from build123d import *

# Parameters (mm, degrees)
EXTRUDE_START   = -3.875
SKETCH_1_R      = 2.225
EXTRUDE_1_DEPTH = 1.6
SKETCH_1_3_R    = 4.255
SKETCH_1_3_R_2  = 2.225
EXTRUDE_2_DEPTH = 3.875


with BuildPart() as part:
    # Эскиз1 → Бобышка-Вытянуть1 (new body)
    with BuildSketch(Plane.XY.offset(EXTRUDE_START)):
        with BuildLine():
            Line((0, 4.045727726), (0, -4.045727726))
            ThreePointArc((0, -4.045727726), (-1.653799143, -4.282252786), (-3.175, -4.972863863))
            ThreePointArc((-3.175, -4.972863863), (-12.25, 0), (-3.175, 4.972863863))
            ThreePointArc((-3.175, 4.972863863), (-1.653799143, 4.282252786), (0, 4.045727726))
        make_face()
        with Locations((-6.35, 0)):
            Circle(SKETCH_1_R, mode=Mode.SUBTRACT)
    extrude(amount=-EXTRUDE_1_DEPTH)

    # Эскиз1<3> → Бобышка-Вытянуть2 (add)
    with BuildSketch(Plane.XY):
        with Locations((-6.35, 0)):
            Circle(SKETCH_1_3_R)
        with Locations((-6.35, 0)):
            Circle(SKETCH_1_3_R_2, mode=Mode.SUBTRACT)
    extrude(amount=-EXTRUDE_2_DEPTH)

    # Зеркальное отражение1: part across plane


with BuildPart() as part_1:
    add(part.part)
    add(part.part.mirror(Plane(origin=(0, 0, 0), x_dir=(0, 0, 1), z_dir=(1, 0, 0))))

    # Зеркальное отражение2: part across plane


with BuildPart() as part_2:
    add(part_1.part)
    add(part_1.part.mirror(Plane.XY))


solid = part_2.part
Geometry: final body of the model. Coordinates: model frame, mm. A direction names the side the tool comes from. Give positions to 0.01 mm unless a question says otherwise; leave off trailing zeros. Write each loop counter-clockwise with the first axis right and the second up, starting at its lowest first coordinate (ties: lowest second). Pieces come first, ordered by that corner, then holes. Notation, with made-up numbers: (-14, 72) - (4, 72) arc R34 cw to (4, 109) - close; hole circle Ø7 at (26.5, 5.25). An arc over 180 degrees is marked (long way). Return JSON: item names as keys, results as strings. Group by question number.
1) Section C-C on z = -0.25. Return the cut outline in (x, y) (3 decimals).
2) Section D-D on y = -2.5. Return the cut outline in (x, z) (3 decimals), plus the area to 3 significant figures.
3) Line query: line 1 (Z direction, x = 3, y = -4.75) (3 decimals); line 2 (Y direction, x = 6.35, z = -0.25) (3 decimals); line 3 (X direction, y = 1.75, z = -2.5). Output: solid intervals per line, ascending.
4) First-contact query: P1, Ø1, axis at x = -2, z = 2, coming from the -Y side; P2, Ø3.5, axis at x = -6.35, y = 0, coming from the -Z side; P3, Ø7, axis at x = 6.35, y = 0, coming from the -Z side (3 decimals); P4, Ø2, axis at x = -7.5, z = 4, coming from the +Y side. Flat tips, straight axial feed; report the tip coordinate or a pass-through.
5) Set-up query: faces 1 (the cylindrical face through (-2.42, -1.63, 0.05)), 2 (the flat face through (0, 0, -5.475)). Return all of +Z, -Z, +X, -X, +Y, -Y with unobstructed straight access to the full face (end or side cutting, diameter ignored); none if empty.
6) Mould query, pull axis Z, two halves, no side actions, for faces 3 (the flat face through (0, 0, 3.875)), 4 (the cylindrical face through (8.12, -1.35, -0.08)), 5 (the flat face through (0, 0, 5.475)). Classes: released by +Z, released by -Z, zero draft, split by the parting line, or undercut.
7) Section A-A on x = -6.35. Return the cut outline in (y, z) (3 decimals), plus the area to 3 significant figures.
8) Section B-B on y = 0. Return the cut outline in (x, z) (3 decimals).
Filled in:
{
 "1": {"outline": "circle Ø8.51 at (-6.35, 0); circle Ø8.51 at (6.35, 0); hole circle Ø4.45 at (-6.35, 0); hole circle Ø4.45 at (6.35, 0)"},
 "2": {"outline": "(-11.694, -5.475) - (11.694, -5.475) - (11.694, -3.875) - (9.793, -3.875) - (9.793, 3.875) - (11.694, 3.875) - (11.694, 5.475) - (-11.694, 5.475) - (-11.694, 3.875) - (-9.793, 3.875) - (-9.793, -3.875) - (-11.694, -3.875) - close; hole (-2.907, -3.875) - (2.907, -3.875) - (2.907, 3.875) - (-2.907, 3.875) - close", "area": "182 mm^2"},
 "3": {"line 1": "z = -5.475 to -3.875, 3.875 to 5.475", "line 2": "y = -4.255 to -2.225, 2.225 to 4.255", "line 3": "x = -10.23 to -7.72, -4.98 to -2.47, 2.47 to 4.98, 7.72 to 10.23"},
 "4": {"P1": "stops at y = -1.81", "P2": "passes through", "P3": "stops at z = -5.475", "P4": "stops at y = 5.9"},
 "5": {"face 1": "none", "face 2": "-Z, +X, -X, +Y, -Y"},
 "6": {"face 3": "undercut", "face 4": "zero draft", "face 5": "released by +Z"},
 "7": {"outline": "(-5.9, -5.475) - (-2.225, -5.475) - (-2.225, 5.475) - (-5.9, 5.475) - (-5.9, 3.875) - (-4.255, 3.875) - (-4.255, -3.875) - (-5.9, -3.875) - close; (2.225, -5.475) - (5.9, -5.475) - (5.9, -3.875) - (4.255, -3.875) - (4.255, 3.875) - (5.9, 3.875) - (5.9, 5.475) - (2.225, 5.475) - close", "area": "55.0 mm^2"},
 "8": {"outline": "(-12.25, -5.475) - (-8.575, -5.475) - (-8.575, 5.475) - (-12.25, 5.475) - (-12.25, 3.875) - (-10.605, 3.875) - (-10.605, -3.875) - (-12.25, -3.875) - close; (-4.125, -5.475) - (4.125, -5.475) - (4.125, 5.475) - (-4.125, 5.475) - close; (8.575, -5.475) - (12.25, -5.475) - (12.25, -3.875) - (10.605, -3.875) - (10.605, 3.875) - (12.25, 3.875) - (12.25, 5.475) - (8.575, 5.475) - close; hole (-2.095, -3.875) - (2.095, -3.875) - (2.095, 3.875) - (-2.095, 3.875) - close"}
}
